```python
from build123d import *

# Parameters (mm, degrees)
BOSS_EXTRUDE1_DEPTH      = 2.54
BOSS_EXTRUDE1_DEPTH_BACK = 2.54
BOSS_EXTRUDE2_DEPTH      = 50.8
BOSS_EXTRUDE2_DEPTH_BACK = 55.88
SKETCH3_W                = 5.08
SKETCH3_H                = 127
BOSS_EXTRUDE3_REACH      = 318.532
SKETCH4_R                = 12.7


with BuildPart() as part:
    # Sketch2 → Boss-Extrude1 (new, two sides: drawn at the far end of the back side and taken through both)
    with BuildSketch(Plane.XY.offset(-BOSS_EXTRUDE1_DEPTH_BACK)):
        with BuildLine():
            Line((-114.3, 0), (-126.238, 0))
            Line((-126.238, 0), (-241.804631128, 70.344905904))
            ThreePointArc((-241.804631128, 70.344905904), (-264.145050484, 93.476275329), (-272.288, 124.586514185))
            Line((-272.288, 124.586514185), (-272.288, 127))
            Line((-272.288, 127), (170.688, 127))
            Line((170.688, 127), (170.688, 124.586514185))
            ThreePointArc((170.688, 124.586514185), (162.545050484, 93.476275329), (140.204631128, 70.344905904))
            Line((140.204631128, 70.344905904), (24.638, 0))
            Line((24.638, 0), (12.7, 0))
            Line((12.7, 0), (12.7, 81.28))
            Line((12.7, 81.28), (-114.3, 81.28))
            Line((-114.3, 81.28), (-114.3, 0))
        make_face()
    extrude(amount=BOSS_EXTRUDE1_DEPTH + BOSS_EXTRUDE1_DEPTH_BACK)

    # Sketch3 → Boss-Extrude2 (add, two sides: drawn at the far end of the back side and taken through both)
    with BuildSketch(Plane.XY.offset(2.54).offset(-BOSS_EXTRUDE2_DEPTH_BACK)):
        with Locations((-116.84, 63.5)):
            Rectangle(SKETCH3_W, SKETCH3_H)
        with Locations((15.24, 63.5)):
            Rectangle(SKETCH3_W, SKETCH3_H)
    extrude(amount=BOSS_EXTRUDE2_DEPTH + BOSS_EXTRUDE2_DEPTH_BACK)

    # Sketch4 → Boss-Extrude3 (add, up to next)
    with BuildSketch(Plane(origin=(-114.3, 0, 0), x_dir=(0, 0, -1), z_dir=(1, 0, 0)), mode=Mode.PRIVATE) as boss_extrude3_sk1:
        with Locations(Location((0, 33.02, 0), (0, 0, 270))):
            Circle(SKETCH4_R)
    boss_extrude3_tool1 = extrude(boss_extrude3_sk1.sketch, amount=BOSS_EXTRUDE3_REACH, mode=Mode.PRIVATE) - part.part
    add(boss_extrude3_tool1.solids().sort_by_distance((-114.3, 33.02, 0))[0])


solid = part.part
```
Work out the finished part from the listing and answer in its coordinate system (mm). A direction names the side the tool comes from. Round coordinates to 2 decimals unless told otherwise and drop trailing zeros. Order: outer loops, then holes, each group sorted by start corner. A loop starts at its lowest first (then second) coordinate and runs counter-clockwise, first axis right, second up.
Q1. A cutting plane is placed at A-A, the plane z = -29.5. Determine the outline of the cut face in (x, y).
Solution:
outline: (-119.38, 0) - (-114.3, 0) - (-114.3, 127) - (-119.38, 127) - close; (12.7, 0) - (17.78, 0) - (17.78, 127) - (12.7, 127) - close
Q2. Given pin 1 Ø2.5 at (x, z) = (-40.5, -1) entering from -Y; pin 2 Ø1 at (y, z) = (86.5, -26) entering from +X; pin 3 Ø10 at (y, z) = (100.5, 39.5) entering from -X, each flat-ended and moving along its own axis, determine where each tip first touches the part or whether it passes through.
Solution:
pin 1: stops at y = 20.32
pin 2: stops at x = 17.78
pin 3: stops at x = -119.38
Q3. A cutting plane is placed at B-B, the plane x = 4. Determine the outline of the cut face in (y, z), then the cut area to 3 significant figures.
Solution:
outline: circle Ø25.4 at (33.02, 0); (81.28, -2.54) - (127, -2.54) - (127, 2.54) - (81.28, 2.54) - close
area: 739 mm2
Q4. A tool of negligible diameter and unlimited length cuts with its end or side. For faces 1 (the flat face through (17.78, 63, 28)), 2 (the flat face through (-119.38, 63, 28)), 3 (the flat face through (17.78, 63, -28)), 4 (the flat face through (-50, 104, -2.54)), from which of +Z, -Z, +X, -X, +Y, -Y can it reach the whole face along a straight path? Write none if from no direction.
Solution:
face 1: +Z, +X, +Y, -Y
face 2: +Z, -X, +Y, -Y
face 3: -Z, +X, +Y, -Y
face 4: -Z, +Y
Q5. A cutting plane is placed at D-D, the plane z = 8. Determine the outline of the cut face in (x, y), then the cut area to 3 significant figures.
Solution:
outline: (-119.38, 0) - (-114.3, 0) - (-114.3, 23.16) - (12.7, 23.16) - (12.7, 0) - (17.78, 0) - (17.78, 127) - (12.7, 127) - (12.7, 42.88) - (-114.3, 42.88) - (-114.3, 127) - (-119.38, 127) - close
area: 3,800 mm2
Q6. The mould has two halves that part along X. Classify faces 5 (the flat face through (-178, 79, -2.54)), 6 (the flat face through (-114.3, 63, -1)), 7 (the flat face through (-119.38, 63, -28)): pulls with the +X half, pulls with the -X half, needs draft (parallel to the pull), parting line crosses it, or undercut.
Solution:
face 5: needs draft
face 6: undercut
face 7: pulls with the -X half
Q7. Find the intervals of material crossed by line 1 along X through (y, z) = (31.5, 46.5); line 2 along Z through (x, y) = (88, 91); line 3 along X through (y, z) = (80, -1), in increasing order.
Solution:
line 1: x = -119.38 to -114.3, 12.7 to 17.78
line 2: z = -2.54 to 2.54
line 3: x = -254 to -114.3, 12.7 to 152.4
Q8. A cutting plane is placed at C-C, the plane y = 63.5. Determine the outline of the cut face in (x, z).
Solution:
outline: (-230.56, -2.54) - (-119.38, -2.54) - (-119.38, -53.34) - (-114.3, -53.34) - (-114.3, 53.34) - (-119.38, 53.34) - (-119.38, 2.54) - (-230.56, 2.54) - close; (12.7, -53.34) - (17.78, -53.34) - (17.78, -2.54) - (128.96, -2.54) - (128.96, 2.54) - (17.78, 2.54) - (17.78, 53.34) - (12.7, 53.34) - close
